from build123d import *

# Parameters (mm, degrees)
F0_R          = 31.75
F1_DEPTH      = 50.8
F1_DEPTH_BACK = 50.8
F3_DEPTH      = 76.2
F5_DEPTH      = 50.8


with BuildPart() as f1:
    # F0 (on Top) → F1 (new body, two sides)
    with BuildSketch(Plane.XY) as f1_sk:
        Circle(F0_R)
    extrude(amount=F1_DEPTH)
    extrude(f1_sk.sketch, amount=-F1_DEPTH_BACK)

    # F2 (on Right) → F3 (join)
    with BuildSketch(Plane.YZ):
        with BuildLine():
            ThreePointArc((1.5875, -31.75), (1.122532, -30.627468), (0, -30.1625))
            ThreePointArc((0, -30.1625), (-1.122532, -32.872532), (1.5875, -31.75))
        make_face()
        with BuildLine():
            ThreePointArc((1.5875, 31.75), (-1.122532, 32.872532), (0, 30.1625))
            ThreePointArc((0, 30.1625), (1.122532, 30.627468), (1.5875, 31.75))
        make_face()
    extrude(amount=F3_DEPTH)

    # F4 (on Right) → F5 (join)
    with BuildSketch(Plane.YZ):
        with BuildLine():
            ThreePointArc((1.5875, 19.05), (-1.122532, 20.172532), (0, 17.4625))
            ThreePointArc((0, 17.4625), (1.122532, 17.927468), (1.5875, 19.05))
        make_face()
        with BuildLine():
            ThreePointArc((1.5875, -19.05), (1.122532, -17.927468), (0, -17.4625))
            ThreePointArc((0, -17.4625), (-1.122532, -20.172532), (1.5875, -19.05))
        make_face()
    extrude(amount=-F5_DEPTH)


solid = f1.part
Part model, mm, in its own coordinate system. Round coordinates to 2 decimals unless told otherwise and drop trailing zeros. Order: outer loops, then holes, each group sorted by start corner. A loop starts at its lowest first (then second) coordinate and runs counter-clockwise, first axis right, second up. Notation, with made-up numbers: (56, 30.5) -> (70, 30.5) arc R5 ccw to (70, 38.5) -> close; hole circle Ø11 at (-20, -35.5). An arc over 180 degrees is marked (long way). Put each result on its own line as item: value.
Q1. Band-saw the part on B-B (z = -41.5). Give the cut face in (x, y).
From the geometry:
outline: circle Ø63.5 at (0, 0)
Q2. Wall check: line 1 (Z direction, x = 33, y = 0); line 2 (X direction, y = -26.5, z = -42.5); line 3 (X direction, y = -0.5, z = -35). Give the ranges that are in metal, low to high. Write a range as [from, to].
From the geometry:
line 1: z = [-33.34, -30.16], [30.16, 33.34]
line 2: x = [-17.49, 17.49]
line 3: x = [-31.75, 31.75]
Q3. Band-saw the part on C-C (y = -15). Give the cut face in (x, z), and give its area (3 significant figures).
From the geometry:
outline: (-27.98, -50.8) -> (27.98, -50.8) -> (27.98, 50.8) -> (-27.98, 50.8) -> close
area: 5,690 mm2
Q4. Pin check, flat tips, straight feed: pin 1 Ø10 at (x, z) = (-3, -16.5) entering from -Y; pin 2 Ø10 at (y, z) = (-8, -12) entering from -X; pin 3 Ø5 at (y, z) = (-7.5, 9.5) entering from +X. Stop position of each tip, or through.
From the geometry:
pin 1: stops at y = -31.75
pin 2: stops at x = -31.61
pin 3: stops at x = 31.35
Q5. Band-saw the part on D-D (x = 8.5). Give the cut face in (y, z), and give its area (3 significant figures).
From the geometry:
outline: (-30.59, -50.8) -> (30.59, -50.8) -> (30.59, 50.8) -> (-30.59, 50.8) -> close
area: 6,220 mm2
